from build123d import *

# Parameters (mm, degrees)
BOSS_EXTRUDE1_DEPTH = 15


with BuildPart() as part:
    # Sketch1 → Boss-Extrude1 (new body)
    with BuildSketch(Plane.XY):
        Polygon((45, 50), (-45, 50), (-65, 20), (-65, 10), (-45, 10), (-45, -20), (-65, -20), (-65, -30), (-25, -50), (25, -50), (65, -30), (65, -20), (45, -20), (45, 10), (65, 10), (65, 20), align=None)
        with BuildLine():
            Line((-5, 30), (5, 30))
            add(Edge.make_bspline(
                [(5, 30), (15, 20), (25, 5), (15, -30), (5, -40)],
                knots=[0, 0, 0, 0, 0, 1, 1, 1, 1, 1], degree=4))
            Line((5, -40), (-5, -40))
            add(Edge.make_bspline(
                [(-5, 30), (-15, 20), (-25, 5), (-15, -30), (-5, -40)],
                knots=[0, 0, 0, 0, 0, 1, 1, 1, 1, 1], degree=4))
        make_face(mode=Mode.SUBTRACT)
    extrude(amount=BOSS_EXTRUDE1_DEPTH)


solid = part.part
Geometry: final body of the model. Coordinates: model frame, mm. A direction names the side the tool comes from. Give positions to 0.01 mm unless a question says otherwise; leave off trailing zeros. Loops run counter-clockwise (first coordinate to the right, second up) from the corner with the lowest first, then second, coordinate; pieces in that order, holes last. Notation, with made-up numbers: (9, -5) - (38, -5) arc R25 cw to (38, 33) - close; hole circle Ø3 at (16.25, 7.25). An arc over 180 degrees is marked (long way). One line per question, with ' | ' between items. Start each with the question number.
(1) Ray query, line 1 (X direction, y = -1.5, z = 3.5); line 2 (Y direction, x = 58, z = 4.5); line 3 (X direction, y = -29.5, z = 7.5). Return the intervals inside material, ascending. Write a range as from..to.
(2) Pull-direction query (Y, two-part tool) for faces 1 (the flat face through (-55, 35, 7)), 2 (the flat face through (-55, 10, 7)), 3 (the flat face through (55, 10, 7)), 4 (the flat face through (65, 15, 7)); classes: released by +Y, released by -Y, zero draft, split by the parting line, or undercut.
(3) Contact query for flat-ended pins moving along their axis: pin 1 (4.5 mm diameter, centred on x = -58.5, z = 4.5, fed in from +Y) (3 decimals); pin 2 (4.5 mm diameter, centred on x = 59.5, z = 7.5, fed in from +Y) (3 decimals); pin 3 (6 mm diameter, centred on y = 3, z = 13, fed in from +X). Output: stop coordinate, or through.
(4) Section query C-C on y = 38.5. Return loops of the section in (x, z), then the cut area to 3 significant figures.
(5) Reachability of faces 5 (the flat face through (55, -20, 7)), 6 (the flat face through (0, -40, 7)), 7 (the flat face through (-45, -5, 7)) from +Z, -Z, +X, -X, +Y, -Y: full face, straight path, thin tool, end or side. Return the list, or none.
(6) Section query A-A on x = 0. Return loops of the section in (y, z).
(7) Section query B-B on x = 28. Return loops of the section in (y, z), then the cut area to 3 significant figures.
The answers:
1) line 1: -45..-17.5, 17.5..45 | line 2: -33.5..-20, 10..30.5 | line 3: -65..-11.53, 11.53..65
2) face 1: released by +Y | face 2: undercut | face 3: undercut | face 4: zero draft
3) pin 1: y = 33.125 | pin 2: y = 31.625 | pin 3: x = 45
4) outline: (-52.67, 0) - (52.67, 0) - (52.67, 15) - (-52.67, 15) - close | area: 1,580 mm2
5) face 5: +Z, -Z, +X | face 6: +Z, -Z | face 7: +Z, -Z, -X
6) outline: (-50, 0) - (-40, 0) - (-40, 15) - (-50, 15) - close; (30, 0) - (50, 0) - (50, 15) - (30, 15) - close
7) outline: (-48.5, 0) - (50, 0) - (50, 15) - (-48.5, 15) - close | area: 1,480 mm2
